The listing builds one solid part. Answer for the finished solid, in the listing's coordinates (mm). Face numbers are marked on the shaded views. A direction names the side the tool comes from. Coordinates: 2 decimals unless noted, no trailing zeros. Order: outer loops, then holes, each group sorted by start corner. A loop starts at its lowest first (then second) coordinate and runs counter-clockwise, first axis right, second up. Notation, with made-up numbers: M 86.25,10 L 138.25,10 A34 cw 138.25,46 Z; hole C 33.25,-38.75 d2. An arc over 180 degrees is marked long. One line per item, written item: value. Start each with the question number.
Q1. Determine the mould class of the marked faces 6, 7, 8 and 9 for opening direction X: pulls with the +X half, pulls with the -X half, needs draft (parallel to the pull), parting line crosses it, or undercut.
Q2. For the marked faces 1, 2, 3, 4 and 5, determine the directions among +Z, -Z, +X, -X, +Y, -Y from which every point of the face is accessible in a straight line to the end or side of a thin tool.
Q3. The part is cut by section C-C on x = 20. Give the vertices of the cut face in (y, z).
Q4. Each of these flat-tipped pins is pushed along its axis until it touches: pin 1 Ø6.5 at (x, y) = (17.5, 30) entering from -Z; pin 2 Ø1.5 at (x, z) = (56.5, 5) entering from -Y; pin 3 Ø2 at (x, y) = (62, 8) entering from +Z. Where does it stop, or does it pass through?
Q5. The part is cut by section A-A on y = 25. Give the vertices of the cut face in (x, z).
Q6. The part is cut by section B-B on z = 6.5. Give the vertices of the cut face in (x, y), then the cut area to 3 significant figures.
Q7. Straight lines are drawn through the part: line 1 along Y through (x, z) = (20, 9.3); line 2 along X through (y, z) = (25, 9.15); line 3 along Y through (x, z) = (20, 4.25). For each, find the intervals that lie inside material, in ascending order. Write a range as [from, to].
Q8. The part is cut by section D-D on z = 1.5. Give the vertices of the cut face in (x, y), then the cut area to 3 significant figures.
Autodesk Fusion 360 part; units mm, degrees
sketch "Top" plane through (0, 0, 0) normal (0, 0, 1) x (1, 0, 0)
  line L0 (0, 0) -> (40, 0)
  line L1 (40, 0) -> (40, 50)
  line L2 (40, 50) -> (0, 50)
  line L3 (0, 50) -> (0, 0)
  circle A0 centre (20, 25) radius 11.2
  circle A1 centre (20, 25) radius 6
  dimension "d6" = 40
  dimension "d7" = 50
  dimension "d11" = 22.4
  dimension "d12" = 25
  dimension "d13" = 20
  dimension "d27" = 12
extrude "Extrude1" add sketch "Top" along normal blind 10 contours L0 L1 L2 L3 | A0 | A1
extrude "Extrude2" cut sketch "Top" along normal blind 8 contours A0 | A1
extrude "Extrude5" cut sketch "Top" along normal blind 110 contours A1
sketch "Sketch5" plane through (0, 0, 0) normal (-1, 0, 0) x (0, -1, 0)
  line L0 (-50, 0) -> (0, 0)
  line L1 (0, 0) -> (0, 10)
  line L2 (0, 10) -> (-50, 10)
  line L3 (-50, 10) -> (-50, 0)
  line L4 (-48, 10) -> (-38, 10)
  line L5 (-38, 10) -> (-38, 0)
  line L6 (-38, 0) -> (-48, 0)
  line L7 (-48, 0) -> (-48, 10)
  dimension "d50" = 10
  dimension "d51" = 10
  dimension "d52" = 2
extrude "Extrude8" add sketch "Sketch5" along normal blind 30 contours L0 L2 L4 L5 L6 L7
sketch "Sketch8" plane through (40, 0, 0) normal (1, 0, 0) x (0, 1, 0)
  line L0 (0, 0) -> (50, 0)
  line L1 (50, 0) -> (50, 10)
  line L2 (50, 10) -> (0, 10)
  line L3 (0, 10) -> (0, 0)
  line L4 (2, 10) -> (12, 10)
  line L5 (12, 10) -> (12, 0)
  line L6 (12, 0) -> (2, 0)
  line L7 (2, 0) -> (2, 10)
  dimension "d72" = 10
  dimension "d73" = 10
  dimension "d74" = 2
extrude "Extrude11" add sketch "Sketch8" along normal blind 30 contours L0 L2 L4 L5 L6 L7
sketch "Sketch10" plane through (0, 0, 10) normal (0, 0, 1) x (-1, 0, 0)
  circle A0 centre (-20, -25) radius 6
  line L0 (0, -50) -> (0, -48)
  line L1 (0, -48) -> (30, -48)
  line L2 (30, -48) -> (30, -38)
  line L3 (30, -38) -> (0, -38)
  line L4 (0, -38) -> (0, 0)
  line L5 (0, 0) -> (-40, 0)
  line L6 (-40, 0) -> (-40, -2)
  line L7 (-40, -2) -> (-70, -2)
  line L8 (-70, -2) -> (-70, -12)
  line L9 (-70, -12) -> (-40, -12)
  line L10 (-40, -12) -> (-40, -50)
  line L11 (-40, -50) -> (0, -50)
  line L12 (20.5049, -40.1716) -> (19.4696, -44.0353)
  line L13 (19.4696, -44.0353) -> (22.2981, -46.8637)
  line L14 (22.2981, -46.8637) -> (26.1618, -45.8284)
  line L15 (26.1618, -45.8284) -> (27.197, -41.9647)
  line L16 (27.197, -41.9647) -> (24.3686, -39.1363)
  line L17 (24.3686, -39.1363) -> (20.5049, -40.1716)
  line L18 (-67.0472, -8.4856) -> (-63.9038, -10.9591)
  line L19 (-63.9038, -10.9591) -> (-60.1898, -9.4736)
  line L20 (-60.1898, -9.4736) -> (-59.6194, -5.5144)
  line L21 (-59.6194, -5.5144) -> (-62.7629, -3.0409)
  line L22 (-62.7629, -3.0409) -> (-66.4768, -4.5264)
  line L23 (-66.4768, -4.5264) -> (-67.0472, -8.4856)
  point P0 (23.3333, -43)
  point P1 (-63.3333, -7)
  dimension "d93" = 4
  dimension "d94" = 5
  dimension "d95" = 6.6667
  dimension "d96" = 4
  dimension "d97" = 6.6667
  dimension "d98" = 5
extrude "Extrude13" cut sketch "Sketch10" against normal blind 5 contours L12 L13 L14 L15 L16 L17 | L18 L19 L20 L21 L22 L23
equation "length = 50 mm"
equation "width = 40 mm"
equation "thickness = 10 mm"
equation "extra = 100 mm"
equation "fit_gap = 0.2 mm"
equation "d6 = width"
equation "d7 = length"
equation "d8 = thickness"
equation "bearing_outer_radius = 11.1 mm"
equation "d11 = ( bearing_outer_radius * 2 ) + fit_gap"
equation "d12 = length / 2"
equation "d13 = width / 2"
equation "d14 = thickness - 2 mm"
equation "bearing_inner_radius = ( 8 mm + 4 mm ) / 2"
equation "d27 = bearing_inner_radius * 2"
equation "d28 = thickness + extra"
equation "rack_rock_bracket_length = 30 mm"
equation "rack_rock_bracket_width = 10 mm"
equation "rack_rock_bracket_big_distance = 2 mm"
equation "d50 = rack_rock_bracket_width"
equation "d51 = rack_rock_bracket_width"
equation "d52 = rack_rock_bracket_big_distance"
equation "d53 = rack_rock_bracket_length"
equation "d72 = rack_rock_bracket_width"
equation "d73 = rack_rock_bracket_width"
equation "d74 = rack_rock_bracket_big_distance"
equation "d75 = rack_rock_bracket_length"
equation "bearing_dowel_radius = 0.8 mm"
equation "bearing_dowel_length = 10 mm"
equation "bearing_dowel_big_distance = 2 mm + bearing_dowel_radius"
equation "bearing_dowel_small_distance = rack_rock_bracket_width / 2"
equation "polygon_dowel_hole_side_length = 4 mm"
equation "polygon_dowel_hole_height = 5 mm"
equation "polygon_dowel_small_distance = thickness / 2"
equation "polygon_dowel_big_distance = polygon_dowel_small_distance + ( polygon_dowel_small_distance / 3 )"
equation "d93 = polygon_dowel_hole_side_length"
equation "d94 = polygon_dowel_small_distance"
equation "d95 = polygon_dowel_big_distance"
equation "d96 = polygon_dowel_hole_side_length"
equation "d97 = polygon_dowel_big_distance"
equation "d98 = polygon_dowel_small_distance"
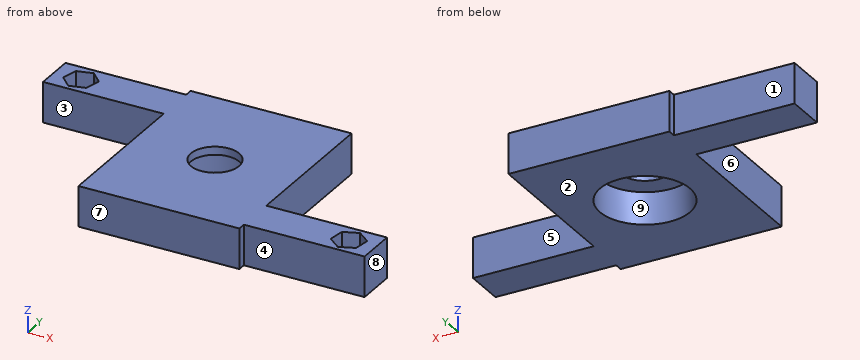
Output:
1. face 6: pulls with the -X half
1. face 7: needs draft
1. face 8: pulls with the +X half
1. face 9: undercut
2. face 1: +Z, -Z, -X, +Y
2. face 2: -Z, +X, -X, +Y, -Y
2. face 3: +Z, -Z, -X, -Y
2. face 4: +Z, -Z, +X, -Y
2. face 5: +Z, -Z, +X, +Y
3. outline: M 0,0 L 13.8,0 L 13.8,8 L 19,8 L 19,10 L 0,10 Z; M 31,8 L 36.2,8 L 36.2,0 L 50,0 L 50,10 L 31,10 Z
4. pin 1: stops at z = 8
4. pin 2: stops at y = 2
4. pin 3: stops at z = 5
5. outline: M 0,0 L 8.8,0 L 8.8,8 L 14,8 L 14,10 L 0,10 Z; M 26,8 L 31.2,8 L 31.2,0 L 40,0 L 40,10 L 26,10 Z
6. outline: M -30,38 L 0,38 L 0,0 L 40,0 L 40,2 L 70,2 L 70,12 L 40,12 L 40,50 L 0,50 L 0,48 L -30,48 Z; hole M -27.2,41.96 L -24.37,39.14 L -20.5,40.17 L -19.47,44.04 L -22.3,46.86 L -26.16,45.83 Z; hole C 20,25 d22.4; hole M 59.62,5.51 L 62.76,3.04 L 66.48,4.53 L 67.05,8.49 L 63.9,10.96 L 60.19,9.47 Z
6. area: 2,120 mm^2
7. line 1: y = [0, 19], [31, 50]
7. line 2: x = [0, 14], [26, 40]
7. line 3: y = [0, 13.8], [36.2, 50]
8. outline: M -30,38 L 0,38 L 0,0 L 40,0 L 40,2 L 70,2 L 70,12 L 40,12 L 40,50 L 0,50 L 0,48 L -30,48 Z; hole C 20,25 d22.4
8. area: 2,210 mm^2
